Check sheet for the modelled part. Datum: model origin and axes. Units: mm. A direction names the side the tool comes from. Coordinates: 2 decimals unless noted, no trailing zeros. Loops run counter-clockwise (first coordinate to the right, second up) from the corner with the lowest first, then second, coordinate; pieces in that order, holes last. Notation, with made-up numbers: M -37,49 L -12,49 A19 cw -12,67 Z; hole C 14.5,25.25 d10. An arc over 180 degrees is marked long. Write each question's results on one line, items separated by ' | '. Start each with the question number.
from build123d import *

# Parameters (mm, degrees)
F0_R      = 24.5
F1_DEPTH  = 255
F2_R      = 24.5
F3_DEPTH  = 14
F4_R      = 14
F6_R      = 26.5
F7_DEPTH  = 13.75
F8_R      = 5
F9_DEPTH  = 85
F10_R     = 15
F11_DEPTH = 200
F13_R     = 12
F14_DEPTH = 18.5


with BuildPart() as f1:
    # F0 (on Top) → F1 (new body)
    with BuildSketch(Plane.XY):
        Circle(F0_R)
    extrude(amount=F1_DEPTH)

    # F2 (on face) → F3 (join)
    with BuildSketch(Plane.XY.offset(255)):
        Circle(F2_R)
    extrude(amount=F3_DEPTH)

    # F4
    f4_edges = [f1.edges().sort_by_distance(p)[0] for p in [
        (-24.5, 0, 269),
    ]]
    fillet(f4_edges, radius=F4_R)

    # F6 (on offset) → F7 (join, symmetric)
    with BuildSketch(Plane.XY.offset(274)):
        Circle(F6_R)
    extrude(amount=F7_DEPTH, both=True)

    # F8 (on Front) → F9 (join)
    with BuildSketch(Plane.XZ):
        with Locations((0, 274)):
            Circle(F8_R)
    extrude(amount=F9_DEPTH)

    # F10 (on Front) → F11 (join)
    with BuildSketch(Plane.XZ):
        with Locations((0, 190)):
            Circle(F10_R)
    extrude(amount=F11_DEPTH)

    # F13 (on offset) → F14 (join)
    with BuildSketch(Plane.XY.offset(190)):
        with Locations((0, -184.25)):
            Circle(F13_R)
    extrude(amount=-F14_DEPTH)


solid = f1.part
1) Section check D-D (y = -147). Enter the section's corners in (x, z), then the cut area to 3 significant figures.
2) Thickness scan on probe 1 along Y at (x, z) = (-1, 227); probe 2 along Y at (x, z) = (-2, 173.5); probe 3 along Z at (x, y) = (2, -25). Record the ranges inside material, lowest first.
3) Gauge pin test, flat ends, axial feed: P1, Ø3, axis at x = 1.5, z = 276, coming from the -Y side; P2, Ø1.5, axis at x = -18, z = 62.5, coming from the +Y side; P3, Ø19, axis at x = -2, y = -188.5, coming from the -Z side. Record the tip position at first contact, or that the pin passes through.
4) Section check B-B (y = -184.25). Enter the section's corners in (x, z), then the cut area to 3 significant figures.
5) Section check C-C (z = 33). Enter the section's corners in (x, y), then the cut area to 3 significant figures.
6) Set-up check for faces 1 (the flat face through (0, -85, 274)), 2 (the flat face through (0, -184, 171.5)), 3 (the flat face through (-16, -18, 260.25)): record each of +Z, -Z, +X, -X, +Y, -Y from which the full face is reachable in a straight line by a thin tool's end or side.
7) Release check for a two-part mould opening along Y. For faces 4 (the cylindrical face through (-0.651, -55.099, 278.957)), 5 (the cylindrical face through (6.45, -174.13, 175.26)), 6 (the flat face through (0, -200, 190)), 7 (the cylindrical face through (-1.953, -108.421, 204.872)) record: +Y half, -Y half, draft (parallel to the pull), parting line (faces both ways), or undercut.
8) Section check A-A (y = -55). Enter the section's corners in (x, z), then the cut area to 3 significant figures.
Return value:
1) outline: C 0,190 d30 | area: 707 mm2
2) probe 1: y = -24.48 to 24.48 | probe 2: y = -196.08 to -172.42, -24.42 to 24.42 | probe 3: z = 175.13 to 204.87, 260.25 to 287.75
3) P1: stops at y = -85 | P2: stops at y = 17.4 | P3: stops at z = 171.5
4) outline: M -12,171.5 L 12,171.5 L 12,181 A15 ccw long -12,181 Z | area: 834 mm2
5) outline: C 0,0 d49 | area: 1,890 mm2
6) face 1: +Z, +X, -X, -Y | face 2: -Z, +X, -X, -Y | face 3: none
7) face 4: draft | face 5: undercut | face 6: -Y half | face 7: undercut
8) outline: C 0,190 d30; C 0,274 d10 | area: 785 mm2
